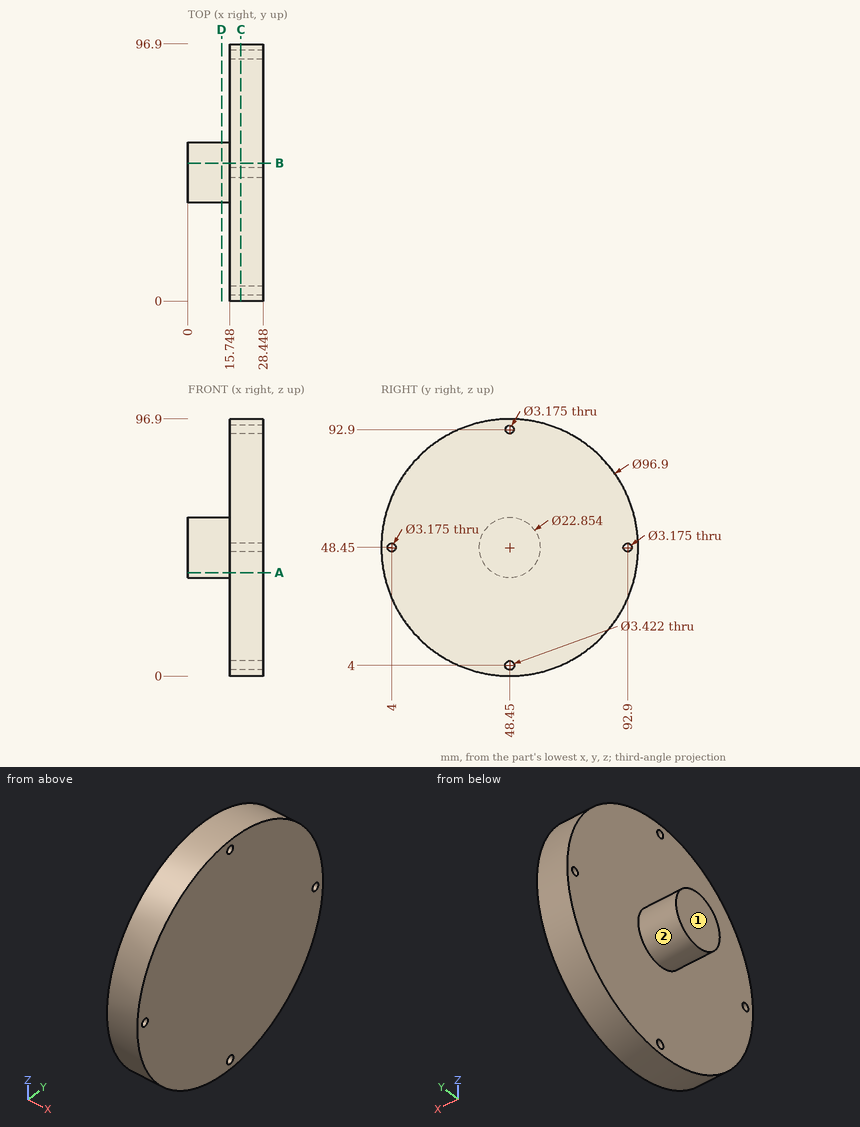
Source: three-view drawing plus pictorial views. Frame: mm from the lowest corner of the part. A direction names the side the tool comes from. Coordinates: 2 decimals unless noted, no trailing zeros. Loops run counter-clockwise (first coordinate to the right, second up) from the corner with the lowest first, then second, coordinate; pieces in that order, holes last. Notation, with made-up numbers: (14.5, 70.5) -> (26.5, 70.5) arc R17 ccw to (26.5, 82.5) -> close; hole circle Ø5 at (0, -35). An arc over 180 degrees is marked (long way). One line per item, written item: value.
(1) Cut plane D-D (x = 12.75). Output: boundary loops of the cut face in (y, z), then the cut area to 3 significant figures.
Answer below:
outline: circle Ø22.85 at (48.45, 48.45)
area: 410 mm2
(2) Pin query (flat end, axial travel): pin 1 Ø2 at (x, y) = (22.5, 56.5) entering from -Z; pin 2 Ø1.5 at (x, y) = (13.5, 14.5) entering from -Z; pin 3 Ø3.5 at (y, z) = (92.9, 48.45) entering from -X; pin 4 Ø5 at (x, y) = (22, 47.5) entering from +Z. Return the tip coordinate at first contact, or that it passes through.
Answer below:
pin 1: stops at z = 0.52
pin 2: passes through
pin 3: stops at x = 15.75
pin 4: stops at z = 96.9
(3) Cut plane B-B (y = 52). Output: boundary loops of the cut face in (x, z), then the cut area to 3 significant figures.
Answer below:
outline: (0, 37.59) -> (15.75, 37.59) -> (15.75, 0.13) -> (28.45, 0.13) -> (28.45, 96.77) -> (15.75, 96.77) -> (15.75, 59.31) -> (0, 59.31) -> close
area: 1,570 mm2
(4) Set-up query: the marked faces 1 and 2. Return all of +Z, -Z, +X, -X, +Y, -Y with unobstructed straight access to the full face (end or side cutting, diameter ignored); none if empty.
Answer below:
face 1: +Z, -Z, -X, +Y, -Y
face 2: -X
(5) Ray query, line 1 along X through (y, z) = (37.5, 21.5); line 2 along Z through (x, y) = (20.75, 47); line 3 along Z through (x, y) = (13, 46). Return the intervals inside material, ascending.
Answer below:
line 1: x = 15.75 to 28.45
line 2: z = 0.02 to 3.09, 4.91 to 92.25, 93.55 to 96.88
line 3: z = 37.29 to 59.61
(6) Cut plane A-A (z = 39). Output: boundary loops of the cut face in (x, y).
Answer below:
outline: (0, 42.03) -> (15.75, 42.03) -> (15.75, 0.93) -> (28.45, 0.93) -> (28.45, 95.97) -> (15.75, 95.97) -> (15.75, 54.87) -> (0, 54.87) -> close
(7) Cut plane C-C (x = 20). Give the number of separate pieces and of enclosed holes in the cut face, then the cut area to 3 significant figures.
Answer below:
separate pieces: 1
enclosed holes: 4
area: 7,340 mm2
